Autodesk Inventor part; units mm, degrees
ref_plane "YZ Plane" through (0, 0, 0) normal (1, 0, 0) x (0, 1, 0)
ref_plane "XZ Plane" through (0, 0, 0) normal (0, 1, 0) x (-1, 0, 0)
ref_plane "XY Plane" through (0, 0, 0) normal (0, 0, 1) x (1, 0, 0)
sketch "Sketch1" plane through (0, 0, 0) normal (0, 0, 1) x (1, 0, 0)
  circle A0 centre (0, 0) radius 7.112
  dimension "d0" = 14.224
extrude "Extrusion1" add sketch "Sketch1" along normal blind 9.652
sketch "Sketch2" plane through (0, 0, 9.652) normal (0, 0, 1) x (1, 0, 0)
  line L0 (2.2997, 3.9555) -> (4.5754, -0.0139)
  line L1 (4.5754, -0.0139) -> (2.2757, -3.9693)
  line L2 (2.2757, -3.9693) -> (-2.2997, -3.9555)
  line L3 (-2.2997, -3.9555) -> (-4.5754, 0.0139)
  line L4 (-4.5754, 0.0139) -> (-2.2757, 3.9693)
  line L5 (-2.2757, 3.9693) -> (2.2997, 3.9555)
  point P0 (0, 0)
  point P1 (0, 0)
  dimension "d3" = 7.9248
extrude "Extrusion2" cut sketch "Sketch2" against normal blind 4.6228
chamfer "Chamfer1" distance 0.508 angle 45 1 edges at (-7.112, 0, 9.652)
sketch "Sketch3" plane through (0, 0, 0) normal (0, 0, -1) x (-1, 0, 0)
  circle A0 centre (0, 0) radius 4.7625
  dimension "d9" = 9.525
extrude "Extrusion3" add sketch "Sketch3" along normal blind 25.4
thread "Thread1"
properties part number "3-8-16 UNC Bolt" material "Stainless Steel"
Source: CAD feature listing. Evaluate the final solid. Frame: model axes, mm. A direction names the side the tool comes from. Coordinates: 2 decimals unless noted, no trailing zeros. Loops run counter-clockwise (first coordinate to the right, second up) from the corner with the lowest first, then second, coordinate; pieces in that order, holes last. Notation, with made-up numbers: (26, 8) - (81, 8) arc R9 cw to (81, 22) - close; hole circle Ø5 at (-33.5, -2.5). An arc over 180 degrees is marked (long way). One line per item, written item: value. Start each with the question number.
1. Set-up query: faces 4 (the cylindrical face through (-1.542, 6.943, 4.508)), 5 (the flat face through (0, 0, 5.029)), 6 (the flat face through (1, -5, 0)). Return all of +Z, -Z, +X, -X, +Y, -Y with unobstructed straight access to the full face (end or side cutting, diameter ignored); none if empty.
2. Section A-A (z = 5.5). Return the cut outline in (x, y).
3. Section C-C (z = -7). Return the cut outline in (x, y) (1 decimal).
4. Section B-B (x = 0). Return the cut outline in (y, z).
5. Mould query, pull axis X, two halves, no side actions, for faces 1 (the flat face through (-0.1, -4.3, 9.652)), 2 (the cylindrical face through (3.78, 2.9, -12.52)), 3 (the flat face through (3.442, -1.964, 7.373)). Classes: pulls with the +X half, pulls with the -X half, needs draft (parallel to the pull), parting line crosses it, or undercut.
6. Ray query, L1, parallel to Z at x = -2, y = -4.75; L2, parallel to Z at x = 3, y = 2.5; L3, parallel to Y at x = 4, z = 7.5. Return the intervals inside material, ascending.
7. Contact query for flat-ended pins moving along their axis: P1, Ø6, axis at x = 4.5, z = -11, coming from the -Y side; P2, Ø2, axis at y = 2, z = -20.5, coming from the +X side; P3, Ø3, axis at x = -2, z = -17.5, coming from the -Y side; P4, Ø6.5, axis at x = 0, y = -1.5, coming from the +Z side. Output: stop coordinate, or through.
Verdict:
1. face 4: +Z, -Z
1. face 5: +Z
1. face 6: -Z
2. outline: circle Ø14.22 at (0, 0); hole (-4.58, 0.01) - (-2.3, -3.96) - (2.28, -3.97) - (4.58, -0.01) - (2.3, 3.96) - (-2.28, 3.97) - close
3. outline: circle Ø9.5 at (0, 0)
4. outline: (-7.11, 0) - (-4.76, 0) - (-4.76, -25.4) - (4.76, -25.4) - (4.76, 0) - (7.11, 0) - (7.11, 9.14) - (6.6, 9.65) - (3.96, 9.65) - (3.96, 5.03) - (-3.96, 5.03) - (-3.96, 9.65) - (-6.6, 9.65) - (-7.11, 9.14) - close
5. face 1: needs draft
5. face 2: parting line crosses it
5. face 3: undercut
6. L1: z = 0 to 9.65
6. L2: z = -25.4 to 5.03
6. L3: y = -5.88 to -1, 0.99 to 5.88
7. P1: stops at y = -4.52
7. P2: stops at x = 4.66
7. P3: stops at y = -4.74
7. P4: stops at z = 9.65
